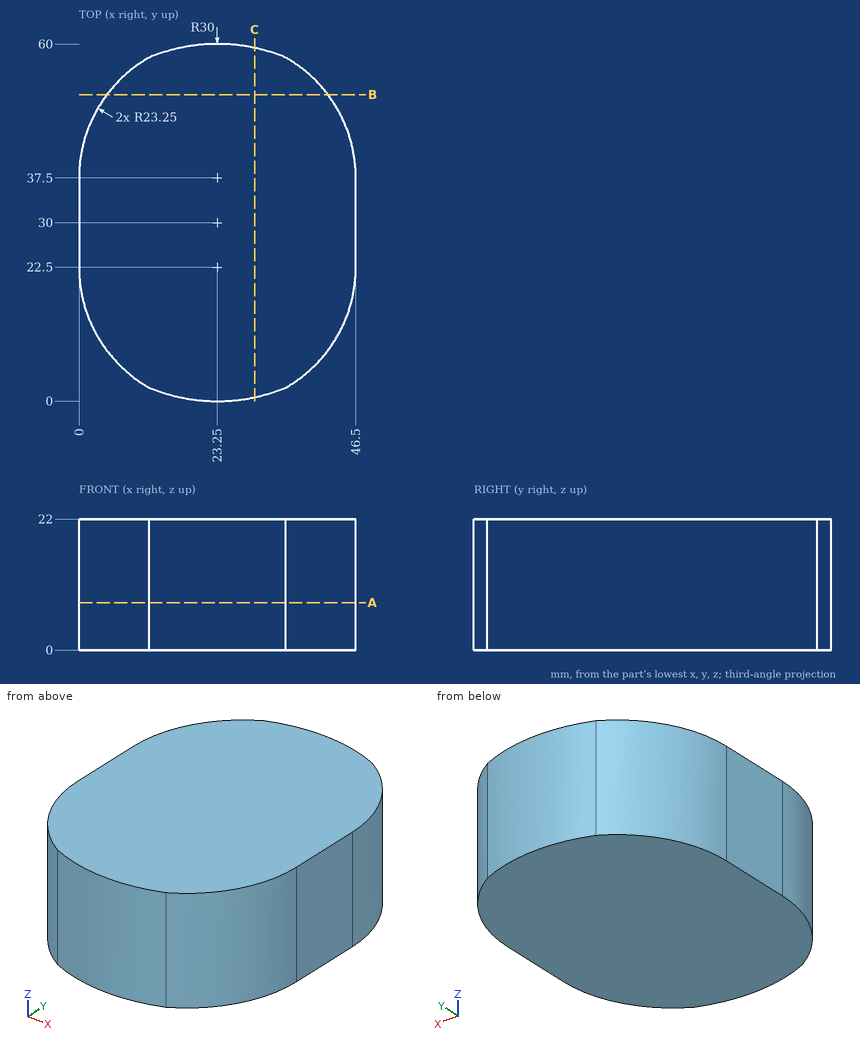
Part print with two shaded views. Sizes in mm from the minimum x, y, z corner. Give positions to 0.01 mm unless a question says otherwise; leave off trailing zeros. Loops run counter-clockwise (first coordinate to the right, second up) from the corner with the lowest first, then second, coordinate; pieces in that order, holes last. Notation, with made-up numbers: (14.25, 8.5) -> (66.25, 8.5) arc R32 cw to (66.25, 37.5) -> close; hole circle Ø4 at (-10.75, -31). An arc over 180 degrees is marked (long way). One line per question, with ' | ' between items.
Q1. Cut at C-C, the plane x = 29.5. Write the cut outline in (y, z), plus the area to 3 significant figures.
Filled sheet:
outline: (0.66, 0) -> (59.34, 0) -> (59.34, 22) -> (0.66, 22) -> close | area: 1,290 mm²
Q2. Drill centre lines: line 1 along Y through (x, z) = (44.5, 11.75); line 2 along Y through (x, z) = (42, 2.5); line 3 along X through (y, z) = (40, 20.5). Where is each one in solid material? Low to high. Write a range as [from, to].
Filled sheet:
line 1: y = [13.07, 46.93] | line 2: y = [8.75, 51.25] | line 3: x = [0.13, 46.37]
Q3. Cut at A-A, the plane z = 8. Write the cut outline in (x, y), plus the area to 3 significant figures.
Filled sheet:
outline: (0, 22.5) arc R23.25 ccw to (11.76, 2.29) arc R30 ccw to (34.74, 2.29) arc R23.25 ccw to (46.5, 22.5) -> (46.5, 37.5) arc R23.25 ccw to (34.74, 57.71) arc R30 ccw to (11.76, 57.71) arc R23.25 ccw to (0, 37.5) -> close | area: 2,370 mm²
Q4. Drop flat-ended pins along their axis: pin 1 (1.5 mm diameter, centred on x = 6, z = 9.5, fed in from +Y); pin 2 (3 mm diameter, centred on x = 22.5, z = 6, fed in from -Y); pin 3 (6 mm diameter, centred on y = 50, z = 18.5, fed in from -X). Give the stop position or say it passes through.
Filled sheet:
pin 1: stops at y = 53.88 | pin 2: stops at y = 0 | pin 3: stops at x = 2.03
Q5. Cut at B-B, the plane y = 51.5. Write the cut outline in (x, z).
Filled sheet:
outline: (4.69, 0) -> (41.81, 0) -> (41.81, 22) -> (4.69, 22) -> close
